Geometry: final body of the model. Coordinates: model frame, mm. Face numbers are marked on the shaded views. A direction names the side the tool comes from. Give positions to 0.01 mm unless a question says otherwise; leave off trailing zeros. Write each loop counter-clockwise with the first axis right and the second up, starting at its lowest first coordinate (ties: lowest second). Pieces come first, ordered by that corner, then holes. Notation, with made-up numbers: (-35.5, 26) -> (-1.5, 26) arc R8 cw to (-1.5, 30) -> close; hole circle Ø2 at (-33.75, 18). An arc over 180 degrees is marked (long way). Use CSV: the item, a comma, the result in double quotes. Start each with the question number.
1) Material intervals for line 1 (X direction, y = 0, z = -3.75); line 2 (X direction, y = -46, z = -0.25); line 3 (X direction, y = -1, z = -4.75), sorted ascending. Write a range as [from, to].
2) Section C-C (x = -0.5). Output: boundary loops of the cut face in (y, z).
3) Contact query for flat-ended pins moving along their axis: P1, Ø4, axis at y = -5.5, z = -2.5, coming from the +X side; P2, Ø1.2, axis at x = 36.5, y = -51.5, coming from the +Z side; P3, Ø4, axis at y = -46.5, z = -4, coming from the -X side. Output: stop coordinate, or through.
4) Section D-D (x = 31.5). Output: boundary loops of the cut face in (y, z).
5) Section B-B (z = -5.5). Count the separate pieces of the cut face and the enclosed holes in it, plus the area to 3 significant figures.
6) Draft query along X for the marked faces 3 and 4. Return one class per face: pulls with the +X half, pulls with the -X half, needs draft (parallel to the pull), parting line crosses it, or undercut.
7) Set-up query: the marked faces 1 and 2. Return all of +Z, -Z, +X, -X, +Y, -Y with unobstructed straight access to the full face (end or side cutting, diameter ignored); none if empty.
8) Section A-A (y = -27). Output: boundary loops of the cut face in (x, z), plus the area to 3 significant figures.
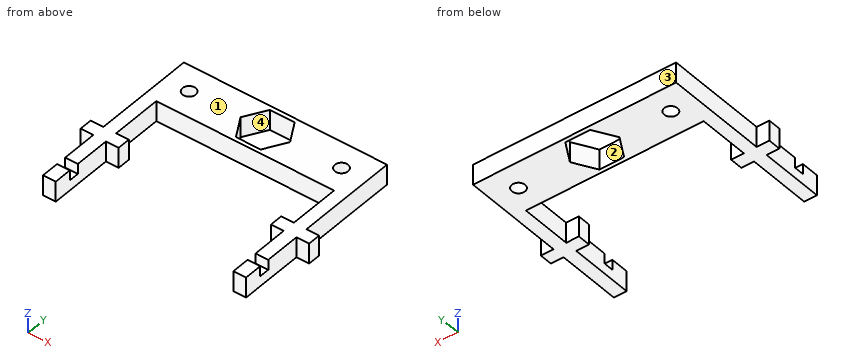
Autodesk Inventor part; units mm, degrees
ref_plane "YZ Plane" through (0, 0, 0) normal (1, 0, 0) x (0, 1, 0)
ref_plane "XZ Plane" through (0, 0, 0) normal (0, 1, 0) x (-1, 0, 0)
ref_plane "XY Plane" through (0, 0, 0) normal (0, 0, 1) x (1, 0, 0)
sketch "Sketch1" plane through (0, 0, 0) normal (0, 0, 1) x (1, 0, 0)
  line L0 (40, -10) -> (-40, -10)
  line L1 (-40, -10) -> (-40, 10)
  line L2 (-40, 10) -> (40, 10)
  line L3 (40, 10) -> (40, -10)
  line L4 (0, -14) -> (0, 14)
  line L5 (40, -10) -> (30, -10)
  line L6 (-56, 0) -> (56, 0)
  circle A0 centre (-0.5449, 0.9437) radius 3.3235
  line L7 (-4.875, -6.5563) -> (-9.2051, 0.9437)
  line L8 (-9.2051, 0.9437) -> (-4.875, 8.4437)
  line L9 (-4.875, 8.4437) -> (3.7853, 8.4437)
  line L10 (3.7853, 8.4437) -> (8.1154, 0.9437)
  line L11 (8.1154, 0.9437) -> (3.7853, -6.5563)
  line L12 (3.7853, -6.5563) -> (-4.875, -6.5563)
  circle A1 centre (-0.5449, 0.9437) radius 3.3235
  line L13 (-4.875, -6.5563) -> (-9.2051, 0.9437)
  line L14 (-9.2051, 0.9437) -> (-4.875, 8.4437)
  line L15 (-4.875, 8.4437) -> (3.7853, 8.4437)
  line L16 (3.7853, 8.4437) -> (8.1154, 0.9437)
  line L17 (8.1154, 0.9437) -> (3.7853, -6.5563)
  line L18 (3.7853, -6.5563) -> (-4.875, -6.5563)
  point P0 (0, 0)
  dimension "d0" = 80
  dimension "d1" = 20
  dimension "d70" = 40
  dimension "d73" = 10
extrude "Extrusion1" add sketch "Sketch1" against normal blind 8
sketch "Sketch3" plane through (0, 0, 0) normal (0, 0, 1) x (1, 0, 0)
  line L0 (0, -14) -> (0, 14)
  line L1 (-56, 0) -> (56, 0)
  line L2 (-4.875, 8.4437) -> (4.875, 8.4437)
  line L3 (4.875, 8.4437) -> (9.75, 0)
  line L4 (9.75, 0) -> (4.875, -8.4437)
  line L5 (4.875, -8.4437) -> (-4.875, -8.4437)
  line L6 (-4.875, -8.4437) -> (-9.75, 0)
  line L7 (-9.75, 0) -> (-4.875, 8.4437)
  point P0 (0, 0)
  point P1 (0, 0)
  dimension "d65" = 19.5
extrude "Extrusion2" cut sketch "Sketch3" against normal blind 10
sketch "Sketch9" plane through (0, 0, -8) normal (0, 0, -1) x (-1, 0, 0)
  circle A0 centre (-30, 0) radius 2.6
  line L0 (0, -14) -> (0, 14)
  line L1 (56, 0) -> (-56, 0)
  circle A1 centre (30, 0) radius 2.6
  dimension "d40" = 5.2
  dimension "d41" = 60
extrude "Extrusion3" cut sketch "Sketch9" against normal through all
sketch "Sketch14" plane through (0, 0, 0) normal (0, 0, 1) x (1, 0, 0)
  circle A0 centre (30, 0) radius 2.6
  circle A1 centre (-30, 0) radius 2.6
  line L0 (-9.75, 0) -> (-4.875, 8.4437)
  line L1 (-4.875, 8.4437) -> (4.875, 8.4437)
  line L2 (4.875, 8.4437) -> (9.75, 0)
  line L3 (9.75, 0) -> (4.875, -8.4437)
  line L4 (4.875, -8.4437) -> (-4.875, -8.4437)
  line L5 (-4.875, -8.4437) -> (-9.75, 0)
  line L6 (40, -10) -> (-40, -10)
  line L7 (40, 10) -> (40, -10)
  line L8 (-40, 10) -> (40, 10)
  line L9 (-40, -10) -> (-40, 10)
  line L10 (-40, -10) -> (-35, -10)
  line L11 (-35, -10) -> (-35, -60)
  line L12 (-35, -60) -> (-40, -60)
  line L13 (-40, -60) -> (-40, -10)
  line L14 (-56, 0) -> (56, 0)
  line L15 (0, -33.313) -> (0, 17.2188)
  line L16 (40, -10) -> (35, -10)
  line L17 (35, -10) -> (35, -60)
  line L18 (35, -60) -> (40, -60)
  line L19 (40, -60) -> (40, -10)
  line L20 (-40, -30) -> (-45, -30)
  line L21 (-45, -30) -> (-45, -35)
  line L22 (-45, -35) -> (-40, -35)
  line L23 (-40, -35) -> (-40, -30)
  line L24 (-35, -30) -> (-30, -30)
  line L25 (-30, -30) -> (-30, -35)
  line L26 (-30, -35) -> (-35, -35)
  line L27 (-35, -35) -> (-35, -30)
  line L28 (40, -30) -> (45, -30)
  line L29 (45, -30) -> (45, -35)
  line L30 (45, -35) -> (40, -35)
  line L31 (40, -35) -> (40, -30)
  line L32 (35, -30) -> (30, -30)
  line L33 (30, -30) -> (30, -35)
  line L34 (30, -35) -> (35, -35)
  line L35 (35, -35) -> (35, -30)
  point P0 (0, 0)
  dimension "d74" = 5
  dimension "d75" = 50
  dimension "d78" = 5
  dimension "d79" = 5
  dimension "d80" = 5
  dimension "d81" = 20
extrude "Extrusion8" add sketch "Sketch14" against normal blind 8 contours L19 L18 L17 L6 | L28 L29 L30 L19 | L17 L34 L33 L32 | L11 L12 L13 L6 | L24 L25 L26 L11 | L13 L22 L21 L20
sketch "Sketch15" plane through (-40, -60, 0) normal (-1, 0, 0) x (0, 0, 1)
  line L0 (0, 25) -> (-8, 25)
  line L1 (-8, 0) -> (-8, 25)
  line L2 (0, 0) -> (-8, 0)
  line L3 (0, 25) -> (0, 0)
  line L4 (0, 70) -> (0, 30)
  line L5 (0, 70) -> (-8, 70)
  line L6 (-8, 30) -> (-8, 70)
  line L7 (0, 30) -> (-8, 30)
  line L8 (0, 25) -> (-8, 25)
  line L9 (0, 30) -> (0, 25)
  line L10 (0, 30) -> (-8, 30)
  line L11 (-8, 25) -> (-8, 30)
  line L12 (0, 25) -> (-8, 25)
  line L13 (0, 11) -> (-4, 11)
  line L14 (-4, 11) -> (-4, 7)
  line L15 (-4, 7) -> (0, 7)
  line L16 (0, 7) -> (0, 11)
  point P0 (0, 60)
  dimension "d84" = 4
  dimension "d85" = 4
  dimension "d89" = 14
extrude "Extrusion9" cut sketch "Sketch15" against normal through all contours L3 L15 L14 L13
properties part number "drieparts_assembly2" material "ABS Plastic"
Answers follow:
1,line 1,"x = [-40, -32.6], [-27.4, -9.75], [9.75, 27.4], [32.6, 40]"
1,line 2,"x = [-40, -35], [35, 40]"
1,line 3,"x = [-40, -32.4], [-27.6, -9.17], [9.17, 27.6], [32.4, 40]"
2,outline,"(-10, -8) -> (-8.44, -8) -> (-8.44, 0) -> (-10, 0) -> close; (8.44, -8) -> (10, -8) -> (10, 0) -> (8.44, 0) -> close"
3,P1,"stops at x = 40"
3,P2,"stops at z = -4"
3,P3,"stops at x = -40"
4,outline,"(-35, -8) -> (-30, -8) -> (-30, 0) -> (-35, 0) -> close; (-10, -8) -> (-2.12, -8) -> (-2.12, 0) -> (-10, 0) -> close; (2.12, -8) -> (10, -8) -> (10, 0) -> (2.12, 0) -> close"
5,separate pieces,"1"
5,enclosed holes,"3"
5,area,"1,910 mm^2"
6,face 3,"needs draft"
6,face 4,"undercut"
7,face 1,"+Z, +X, -X, +Y, -Y"
7,face 2,"+Z, -Z"
8,outline,"(-40, -8) -> (-35, -8) -> (-35, 0) -> (-40, 0) -> close; (35, -8) -> (40, -8) -> (40, 0) -> (35, 0) -> close"
8,area,"80.0 mm^2"
